```python
from build123d import *

# Parameters (mm, degrees)
BOSS_EXTRUDE1_DEPTH = 0.125
SKETCH3_W           = 0.125
SKETCH3_H           = 15.25
BOSS_EXTRUDE2_DEPTH = 15.766908
SKETCH4_W           = 15.766907998
SKETCH4_H           = 0.125
BOSS_EXTRUDE3_DEPTH = 2.5
CUT_EXTRUDE1_DEPTH  = 2.5
FILLET1_R           = 0.4
FILLET2_R           = 0.5
FILLET3_R           = 0.5
FILLET4_R           = 2
FILLET5_R           = 2
FILLET6_R           = 0.4
CUT_EXTRUDE2_START  = -17.75
CUT_EXTRUDE2_DEPTH  = 17.75
FILLET7_R           = 2


with BuildPart() as part:
    # Sketch2 → Boss-Extrude1 (new body)
    with BuildSketch(Plane(origin=(0, 0, 0), x_dir=(1, 0, 0), z_dir=(0, 1, 0))):
        with BuildLine():
            Line((-7.883453999, 0), (-5.5, 0))
            ThreePointArc((-5.5, 0), (0, -5.5), (5.5, 0))
            Line((5.5, 0), (7.883453999, 0))
            Line((7.883453999, 0), (7.883453999, -9))
            Line((7.883453999, -9), (-7.883453999, -9))
            Line((-7.883453999, -9), (-7.883453999, 0))
        make_face()
    extrude(amount=BOSS_EXTRUDE1_DEPTH)

    # Sketch3 → Boss-Extrude2 (add)
    with BuildSketch(Plane(origin=(7.883453999, 0, 0), x_dir=(0, 0, -1), z_dir=(1, 0, 0))):
        with Locations((-9.0625, -7.5)):
            Rectangle(SKETCH3_W, SKETCH3_H)
    extrude(amount=-BOSS_EXTRUDE2_DEPTH)

    # Sketch4 → Boss-Extrude3 (add)
    with BuildSketch(Plane.XZ.offset(15.125)):
        with Locations((0, 9.0625)):
            Rectangle(SKETCH4_W, SKETCH4_H)
    extrude(amount=BOSS_EXTRUDE3_DEPTH)

    # Sketch5 → Cut-Extrude1 (cut)
    with BuildSketch(Plane.XY.offset(9.125)):
        with BuildLine():
            Line((-3.156922186, -14.375), (2.843077814, -14.375))
            ThreePointArc((2.843077814, -14.375), (4.093077814, -15.625), (2.843077814, -16.875))
            Line((2.843077814, -16.875), (-3.156922186, -16.875))
            ThreePointArc((-3.156922186, -16.875), (-4.406922186, -15.625), (-3.156922186, -14.375))
        make_face()
    extrude(amount=-CUT_EXTRUDE1_DEPTH, mode=Mode.SUBTRACT)

    # Mirror1: part across plane


with BuildPart() as part_1:
    add(part.part)
    add(part.part.mirror(Plane(origin=(5.5, 0.125, 0), x_dir=(1, 0, 0), z_dir=(0, 0, 1))))

    # Fillet1
    fillet1_edges = [part_1.edges().sort_by_distance(p)[0] for p in [
        (-1e-09, 0.125, 9.125),
    ]]
    fillet(fillet1_edges, radius=FILLET1_R)

    # Fillet2
    fillet2_edges = [part_1.edges().sort_by_distance(p)[0] for p in [
        (0, 0, 9),
    ]]
    fillet(fillet2_edges, radius=FILLET2_R)

    # Fillet3
    fillet3_edges = [part_1.edges().sort_by_distance(p)[0] for p in [
        (0, 0, -9),
    ]]
    fillet(fillet3_edges, radius=FILLET3_R)

    # Fillet4
    fillet4_edges = [part_1.edges().sort_by_distance(p)[0] for p in [
        (7.883453999, -17.625, 9.0625),
        (-7.883453999, -17.625, 9.0625),
    ]]
    fillet(fillet4_edges, radius=FILLET4_R)

    # Fillet5
    fillet5_edges = [part_1.edges().sort_by_distance(p)[0] for p in [
        (7.883453999, -17.625, -9.0625),
        (-7.883453999, -17.625, -9.0625),
    ]]
    fillet(fillet5_edges, radius=FILLET5_R)

    # Fillet6
    fillet6_edges = [part_1.edges().sort_by_distance(p)[0] for p in [
        (-1e-09, 0.125, -9.125),
    ]]
    fillet(fillet6_edges, radius=FILLET6_R)

    # Sketch6 → Cut-Extrude2 (cut)
    with BuildSketch(Plane(origin=(0, 0.125, 0), x_dir=(1, 0, 0), z_dir=(0, 1, 0)).offset(CUT_EXTRUDE2_START)):
        Polygon((7.883453999, -8.725), (5, -8.725), (5, -13.174899539), (11.0971106, -13.174899539), (11.0971106, 15.116605335), (5, 15.116605335), (5, 8.725), (7.883453999, 8.725), align=None)
        Polygon((-5, -13.174899539), (-5, -8.725), (-7.883453999, -8.725), (-7.883453999, 8.725), (-5, 8.725), (-5, 15.116605335), (-11.0971106, 15.116605335), (-11.0971106, -13.174899539), align=None)
        with BuildLine():
            Line((5, -5.590169944), (5, -8.725))
            Line((5, -8.725), (7.883453999, -8.725))
            Line((7.883453999, -8.725), (7.883453999, 8.725))
            Line((7.883453999, 8.725), (5, 8.725))
            Line((5, 8.725), (5, 5.590169944))
            ThreePointArc((5, 5.590169944), (6.846531969, 3.061862178), (7.5, 0))
            ThreePointArc((7.5, 0), (6.846531969, -3.061862178), (5, -5.590169944))
        make_face()
        with BuildLine():
            Line((-7.883453999, -8.725), (-5, -8.725))
            Line((-5, -8.725), (-5, -5.590169944))
            ThreePointArc((-5, -5.590169944), (-7.5, 0), (-5, 5.590169944))
            Line((-5, 5.590169944), (-5, 8.725))
            Line((-5, 8.725), (-7.883453999, 8.725))
            Line((-7.883453999, 8.725), (-7.883453999, -8.725))
        make_face()
    extrude(amount=CUT_EXTRUDE2_DEPTH, mode=Mode.SUBTRACT)

    # Fillet7
    fillet7_edges = [part_1.edges().sort_by_distance(p)[0] for p in [
        (5, -17.625, 9.0625),
        (5, -17.625, -9.0625),
        (-5, -17.625, 9.0625),
        (-5, -17.625, -9.0625),
    ]]
    fillet(fillet7_edges, radius=FILLET7_R)


solid = part_1.part
```
Work out the finished part from the listing and answer in its coordinate system (mm). Coordinates: 2 decimals unless noted, no trailing zeros. Loops run counter-clockwise (first coordinate to the right, second up) from the corner with the lowest first, then second, coordinate; pieces in that order, holes last. Notation, with made-up numbers: (65, 20) -> (121, 20) arc R18 ccw to (121, 42) -> close; hole circle Ø4 at (57, -7.75). An arc over 180 degrees is marked (long way). Answer as CSV lines item,"result".
Q1. The part is cut by section C-C on z = -5. Write down the section's boundary in (x, y) (3 decimals).
Findings:
outline,"(-5.59, 0) -> (-2.291, 0) -> (-2.291, 0.125) -> (-5.59, 0.125) -> close; (2.291, 0) -> (5.59, 0) -> (5.59, 0.125) -> (2.291, 0.125) -> close"
Q2. The part is cut by section B-B on x = 0. Write down the section's boundary in (y, z) (3 decimals).
Findings:
outline,"(-17.625, -9.125) -> (-16.875, -9.125) -> (-16.875, -9) -> (-17.625, -9) -> close; (-17.625, 9) -> (-16.875, 9) -> (-16.875, 9.125) -> (-17.625, 9.125) -> close; (-14.375, -9.125) -> (-0.275, -9.125) arc R0.4 ccw to (0.125, -8.725) -> (0.125, -5.5) -> (0, -5.5) -> (0, -8.5) arc R0.5 cw to (-0.5, -9) -> (-14.375, -9) -> close; (-14.375, 9) -> (-0.5, 9) arc R0.5 cw to (0, 8.5) -> (0, 5.5) -> (0.125, 5.5) -> (0.125, 8.725) arc R0.4 ccw to (-0.275, 9.125) -> (-14.375, 9.125) -> close"
Q3. Each of these flat-tipped pins is pushed along its axis until it touches: pin 1 (1.8 mm diameter, centred on y = -6, z = -8, fed in from -X); pin 2 (2 mm diameter, centred on x = -4.5, z = 5.5, fed in from -Y); pin 3 (4 mm diameter, centred on y = -5.5, z = -8, fed in from +X). Where does it stop, or does it pass through?
Findings:
pin 1,"passes through"
pin 2,"stops at y = 0"
pin 3,"stops at x = 5"
Q4. The part is cut by section A-A on y = -13.5. Write down the section's boundary in (x, z) (3 decimals), and give its area (3 significant figures).
Findings:
outline,"(-5, -9.125) -> (5, -9.125) -> (5, -9) -> (-5, -9) -> close; (-5, 9) -> (5, 9) -> (5, 9.125) -> (-5, 9.125) -> close"
area,"2.50 mm²"
Q5. The part is cut by section D-D on x = 4.75. Write down the section's boundary in (y, z) (3 decimals).
Findings:
outline,"(-16.593, -9.125) -> (-0.275, -9.125) arc R0.4 ccw to (0.125, -8.725) -> (0.125, -2.773) -> (0, -2.773) -> (0, -8.5) arc R0.5 cw to (-0.5, -9) -> (-16.593, -9) -> close; (-16.593, 9) -> (-0.5, 9) arc R0.5 cw to (0, 8.5) -> (0, 2.773) -> (0.125, 2.773) -> (0.125, 8.725) arc R0.4 ccw to (-0.275, 9.125) -> (-16.593, 9.125) -> close"
